Input: dimensioned drawing with shaded views. Units: mm. Origin: part minimum x, y, z. Round coordinates to 2 decimals unless told otherwise and drop trailing zeros. Loops run counter-clockwise (first coordinate to the right, second up) from the corner with the lowest first, then second, coordinate; pieces in that order, holes last. Notation, with made-up numbers: (33.25, -17.5) - (51.25, -17.5) arc R28 cw to (51.25, 6.5) - close; hole circle Ø9 at (66, 30). An arc over 180 degrees is marked (long way). One line per question, with ' | ' between items. Start each with the question number.
1. Cut plane B-B (x = 175). Return loops of the section in (y, z).
2. Ray query, line 1 (Y direction, x = 179, z = 2.5) (1 decimal); line 2 (X direction, y = 211, z = 3); line 3 (Y direction, x = 198, z = 1.55). Return the intervals inside material, ascending.
3. Cut plane C-C (z = 2.05). Return loops of the section in (x, y) (1 decimal), then the cut area to 3 significant figures.
4. Pin query (flat end, axial travel): pin 1 (1 mm diameter, centred on y = 206, z = 1.5, fed in from +X); pin 2 (3 mm diameter, centred on y = 41, z = 1, fed in from +X); pin 3 (2 mm diameter, centred on y = 190.5, z = 4, fed in from +X). Return the tip coordinate at first contact, or that it passes through.
5. Cut plane D-D (x = 115.5). Return loops of the section in (y, z) (1 decimal).
6. Cut plane A-A (y = 175). Return loops of the section in (x, z), then the cut area to 3 significant figures.
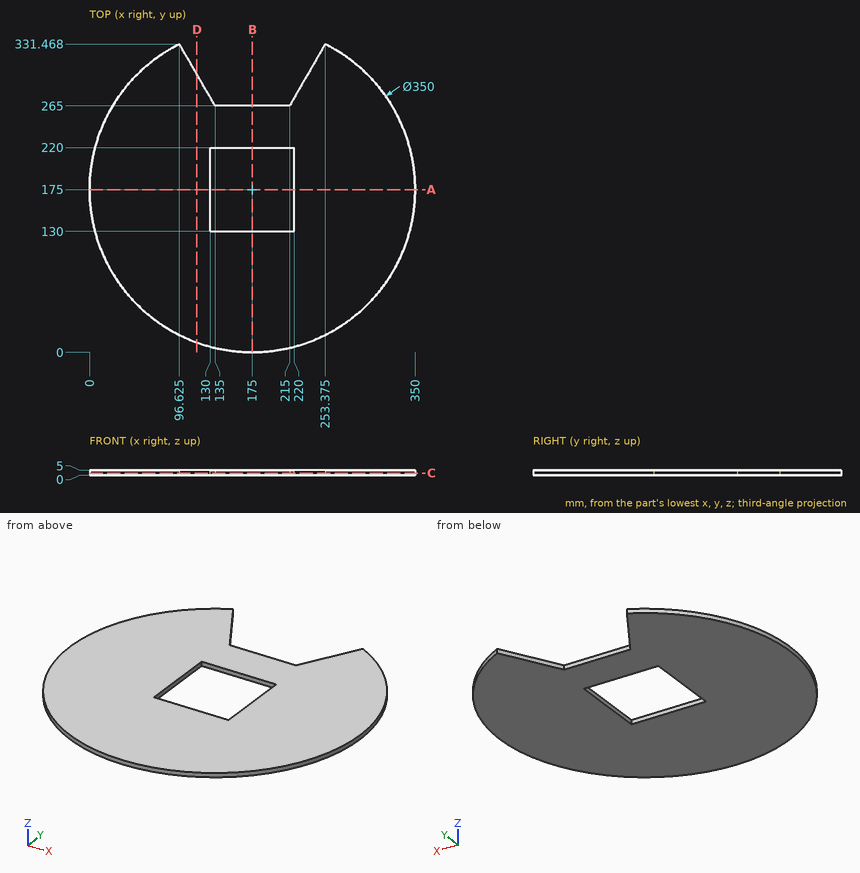
Answers follow:
1) outline: (0, 0) - (130, 0) - (130, 5) - (0, 5) - close; (220, 0) - (265, 0) - (265, 5) - (220, 5) - close
2) line 1: y = 0 to 130, 220 to 265 | line 2: x = 3.74 to 130, 220 to 346.26 | line 3: y = 1.52 to 130, 220 to 265
3) outline: (96.6, 331.5) arc R175 ccw (long way) to (253.4, 331.5) - (215, 265) - (135, 265) - close; hole (130, 130) - (220, 130) - (220, 220) - (130, 220) - close | area: 78,300 mm2
4) pin 1: stops at x = 347.32 | pin 2: stops at x = 289.32 | pin 3: stops at x = 349.4
5) outline: (10.4, 0) - (298.8, 0) - (298.8, 5) - (10.4, 5) - close
6) outline: (0, 0) - (130, 0) - (130, 5) - (0, 5) - close; (220, 0) - (350, 0) - (350, 5) - (220, 5) - close | area: 1,300 mm2
